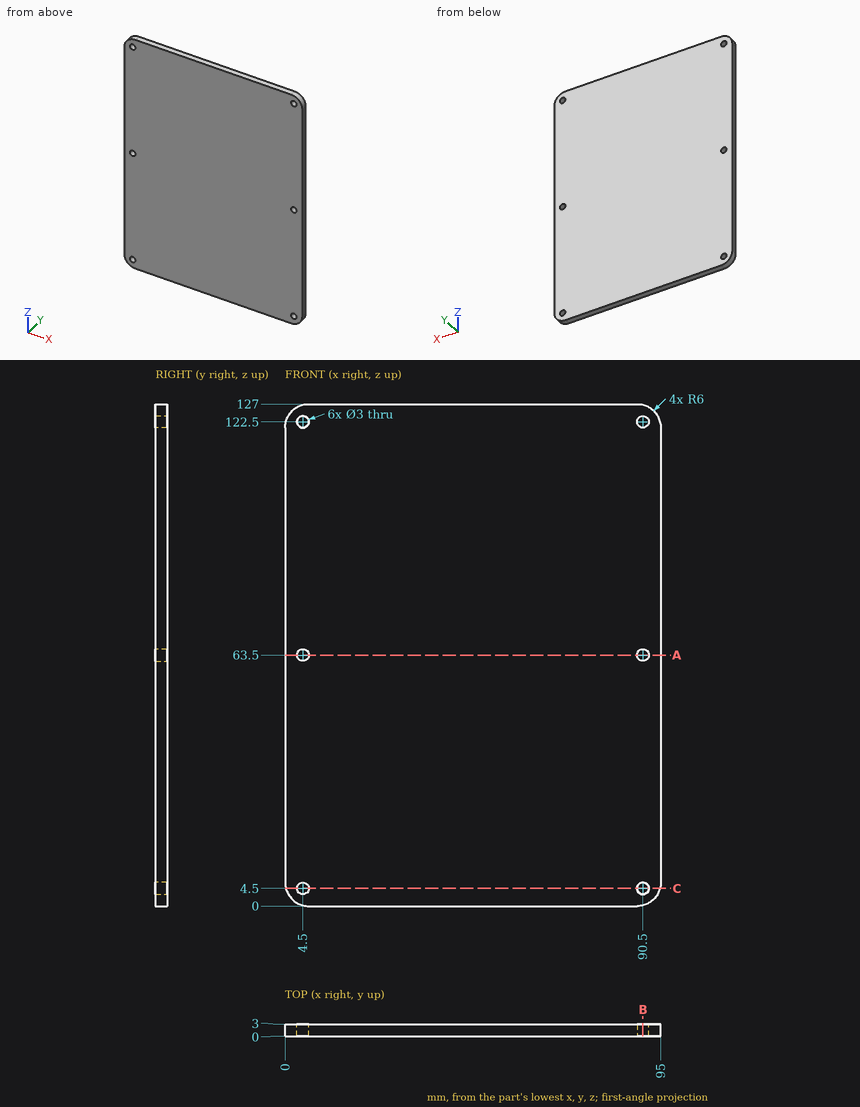
The drawing under review shows one solid part. Ordinate dimensions are in mm from its lowest x, y, z. Give positions to 0.01 mm unless a question says otherwise; leave off trailing zeros. Order: outer loops, then holes, each group sorted by start corner. A loop starts at its lowest first (then second) coordinate and runs counter-clockwise, first axis right, second up. Notation, with made-up numbers: M -38.75,23 L -19.75,23 A16 cw -19.75,48 Z; hole C 0.5,-29.75 d8. An arc over 180 degrees is marked long. Answer in a Markdown table with one row per item. Add a question column.
1. Add section C-C on z = 4.5. State the section outline as (x, y) points, plus the area to 3 significant figures.
2. Add section B-B on x = 90.5. State the section outline as (y, z) points, plus the area to 3 significant figures.
3. Add section A-A on z = 63.5. State the section outline as (x, y) points, plus the area to 3 significant figures.
4. To check wall thickness, follow line 1 along X through (y, z) = (1, 4.5); line 2 along Z through (x, y) = (90.5, 0.9); line 3 along Z through (x, y) = (5, 1.25). State the ranges of each line that lie inside material, in increasing order.
The answers:
| question | item | result |
|---|---|---|
| 1 | outline | M 0.19,0 L 3,0 L 3,3 L 0.19,3 Z; M 6,0 L 89,0 L 89,3 L 6,3 Z; M 92,0 L 94.81,0 L 94.81,3 L 92,3 Z |
| 1 | area | 266 mm2 |
| 2 | outline | M 0,0.19 L 3,0.19 L 3,3 L 0,3 Z; M 0,6 L 3,6 L 3,62 L 0,62 Z; M 0,65 L 3,65 L 3,121 L 0,121 Z; M 0,124 L 3,124 L 3,126.81 L 0,126.81 Z |
| 2 | area | 353 mm2 |
| 3 | outline | M 0,0 L 3,0 L 3,3 L 0,3 Z; M 6,0 L 89,0 L 89,3 L 6,3 Z; M 92,0 L 95,0 L 95,3 L 92,3 Z |
| 3 | area | 267 mm2 |
| 4 | line 1 | 0.19 to 3, 6 to 89, 92 to 94.81 |
| 4 | line 2 | 0.19 to 3, 6 to 62, 65 to 121, 124 to 126.81 |
| 4 | line 3 | 0.08 to 3.09, 5.91 to 62.09, 64.91 to 121.09, 123.91 to 126.92 |
